Print and shaded views of the part. All mm, measured from the part's lowest x, y and z. Give positions to 0.01 mm unless a question says otherwise; leave off trailing zeros. Write each loop counter-clockwise with the first axis right and the second up, starting at its lowest first coordinate (ties: lowest second). Pieces come first, ordered by that corner, then holes. Notation, with made-up numbers: (7, 43) -> (38, 43) arc R26 cw to (38, 66) -> close; hole circle Ø6 at (20, 56). An arc over 180 degrees is marked (long way). Put each result on its own line as item: value.
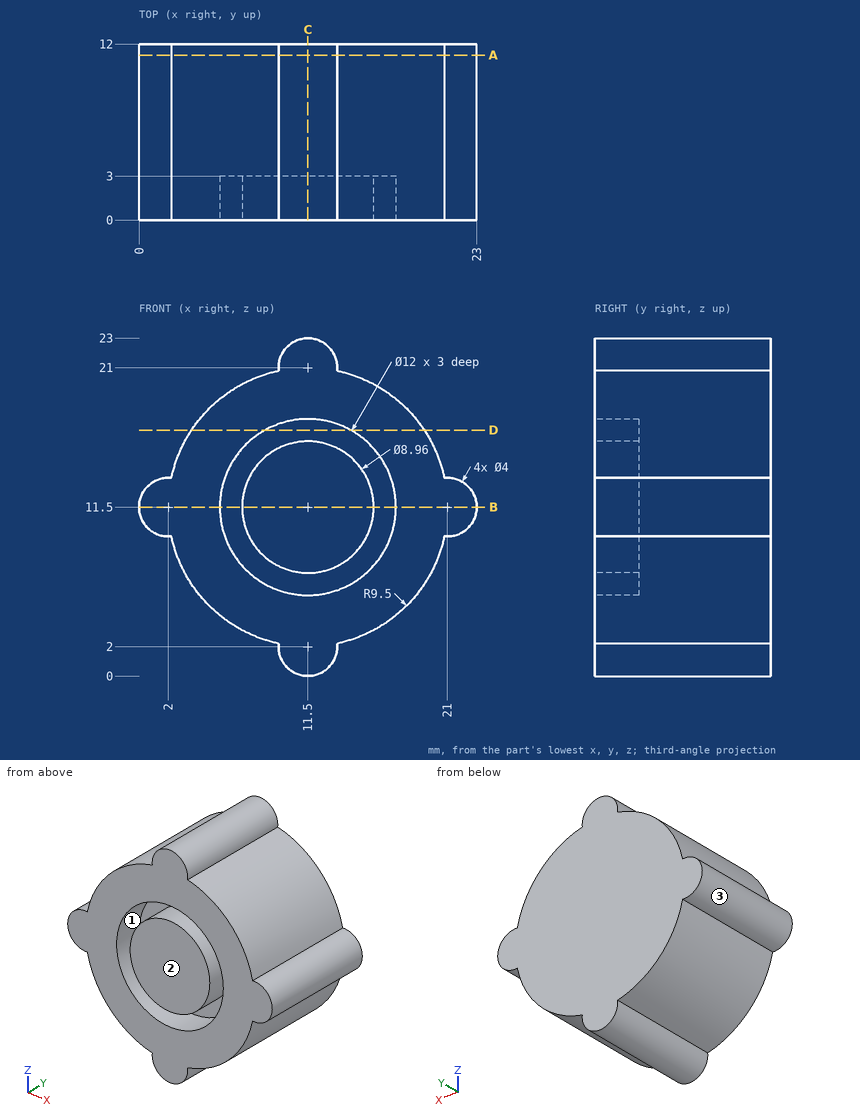
1) Wall check: L1, parallel to Z at x = 11.5, y = 2.1; L2, parallel to Y at x = 15, z = 6.75; L3, parallel to X at y = 1.75, z = 11.75. Give the ranges that are in metal, low to high.
Filled sheet:
L1: 0 to 5.5, 7.02 to 15.98, 17.5 to 23
L2: 3 to 12
L3: 0.02 to 5.51, 7.03 to 15.97, 17.49 to 22.98
2) Slice it at A-A (y = 11.25). Write the cut outline in (x, z), plus the area to 3 significant figures.
Filled sheet:
outline: (2.21, 9.51) arc R9.5 ccw to (9.51, 2.21) arc R2 ccw (long way) to (13.49, 2.21) arc R9.5 ccw to (20.79, 9.51) arc R2 ccw (long way) to (20.79, 13.49) arc R9.5 ccw to (13.49, 20.79) arc R2 ccw (long way) to (9.51, 20.79) arc R9.5 ccw to (2.21, 13.49) arc R2 ccw (long way) to start
area: 310 mm2
3) Slice it at B-B (z = 11.5). Write the cut outline in (x, y), plus the area to 3 significant figures.
Filled sheet:
outline: (0, 0) -> (5.5, 0) -> (5.5, 3) -> (7.02, 3) -> (7.02, 0) -> (15.98, 0) -> (15.98, 3) -> (17.5, 3) -> (17.5, 0) -> (23, 0) -> (23, 12) -> (0, 12) -> close
area: 267 mm2
4) Slice it at D-D (z = 16.75). Write the cut outline in (x, y), plus the area to 3 significant figures.
Filled sheet:
outline: (3.58, 0) -> (8.6, 0) -> (8.6, 3) -> (14.4, 3) -> (14.4, 0) -> (19.42, 0) -> (19.42, 12) -> (3.58, 12) -> close
area: 173 mm2
5) Pin check, flat tips, straight feed: pin 1 (2 mm diameter, centred on x = 4, z = 19.5, fed in from +Y); pin 2 (2 mm diameter, centred on y = 4, z = 18, fed in from -X); pin 3 (5 mm diameter, centred on y = 1.5, z = 17, fed in from +X); pin 4 (1 mm diameter, centred on y = 2.5, z = 8.5, fed in from -X). Stop position of each tip, or through.
Filled sheet:
pin 1: through
pin 2: x = 3.75
pin 3: x = 20.51
pin 4: x = 2.33
6) Pull direction Z, two halves, no side cores. Call the marked faces 1, 2 and 3: released by +Z, released by -Z, zero draft, split by the parting line, or undercut.
Filled sheet:
face 1: undercut
face 2: zero draft
face 3: split by the parting line
7) Slice it at C-C (x = 11.5). Write the cut outline in (y, z).
Filled sheet:
outline: (0, 0) -> (12, 0) -> (12, 23) -> (0, 23) -> (0, 17.5) -> (3, 17.5) -> (3, 15.98) -> (0, 15.98) -> (0, 7.02) -> (3, 7.02) -> (3, 5.5) -> (0, 5.5) -> close
